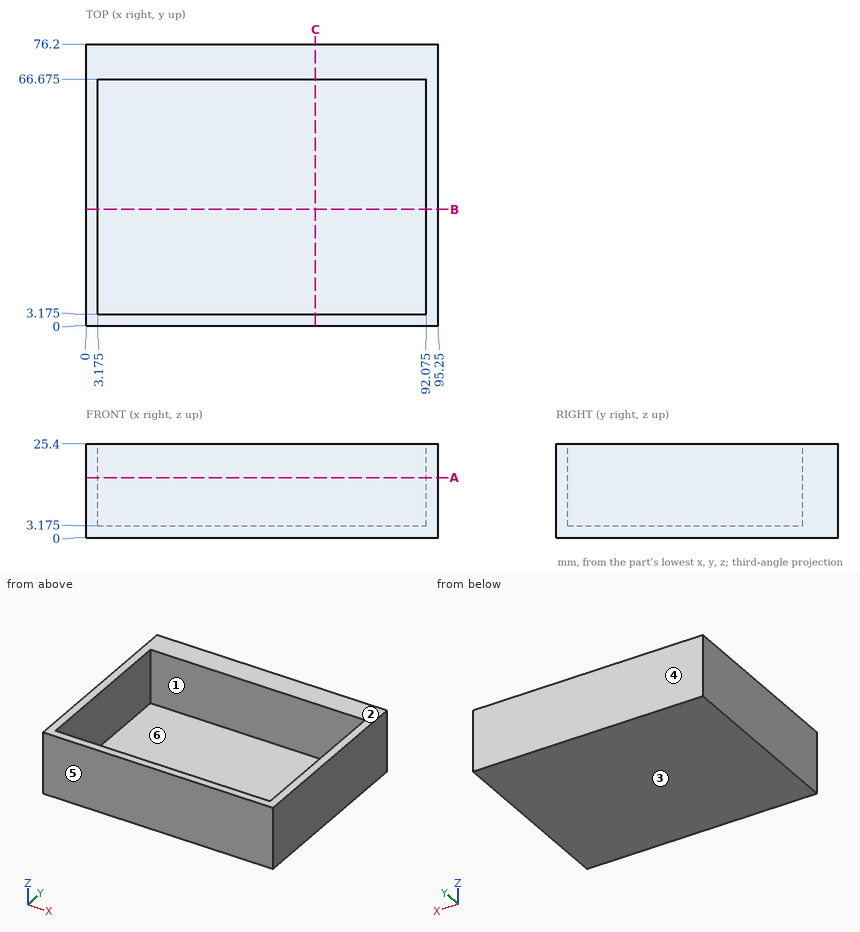
Can you work these out from the drawing? Everything is in mm from the part's minimum corner. A direction names the side the tool comes from. Round coordinates to 2 decimals unless told otherwise and drop trailing zeros. Loops run counter-clockwise (first coordinate to the right, second up) from the corner with the lowest first, then second, coordinate; pieces in that order, holes last. Notation, with made-up numbers: (20, 57) - (57, 57) arc R23 ccw to (57, 71) - close; hole circle Ø4 at (11, 15.25). An arc over 180 degrees is marked (long way). Answer as CSV lines item,"result".
1. I want a section at A-A on z = 16.25. List the corners of the cut face in (x, y) for me (3 decimals), then the cut area to 3 significant figures.
Filled in:
outline,"(0, 0) - (95.25, 0) - (95.25, 76.2) - (0, 76.2) - close; hole (3.175, 3.175) - (92.075, 3.175) - (92.075, 66.675) - (3.175, 66.675) - close"
area,"1,610 mm^2"
2. Please list where these lines run through material, in increasing order: line 1 along X through (y, z) = (5, 13) (3 decimals); line 2 along Y through (x, z) = (57, 5.25) (3 decimals); line 3 along Z through (x, y) = (87, 51) (3 decimals). Write a range as [from, to].
Filled in:
line 1,"x = [0, 3.175], [92.075, 95.25]"
line 2,"y = [0, 3.175], [66.675, 76.2]"
line 3,"z = [0, 3.175]"
3. On a 3-axis mill with a long thin cutter (end or side, diameter ignored), from which of +Z, -Z, +X, -X, +Y, -Y can I reach the whole of each face in a straight line? I mean the marked faces 1 and 2. Say none if no direction works.
Filled in:
face 1,"+Z"
face 2,"+Z, +X, -X, +Y, -Y"
4. I want a section at B-B on y = 31.5. List the corners of the cut face in (x, z) for me (3 decimals), then the cut area to 3 significant figures.
Filled in:
outline,"(0, 0) - (95.25, 0) - (95.25, 25.4) - (92.075, 25.4) - (92.075, 3.175) - (3.175, 3.175) - (3.175, 25.4) - (0, 25.4) - close"
area,"444 mm^2"
5. I want a section at C-C on x = 62. List the corners of the cut face in (y, z) for me (3 decimals).
Filled in:
outline,"(0, 0) - (76.2, 0) - (76.2, 25.4) - (66.675, 25.4) - (66.675, 3.175) - (3.175, 3.175) - (3.175, 25.4) - (0, 25.4) - close"
6. For pin 1 Ø8 at (x, y) = (45.5, 40) entering from +Z (3 decimals); pin 2 Ø2 at (x, z) = (70, 9) entering from -Y, each with a flat end and sliding along its axis, tell me the tip position at first contact or that it passes through.
Filled in:
pin 1,"stops at z = 3.175"
pin 2,"stops at y = 0"
7. We'd pull the mould along Y, two halves only. Please class the marked faces 3, 4, 5 and 6: +Y half, -Y half, draft (parallel to the pull), parting line (faces both ways), or undercut.
Filled in:
face 3,"draft"
face 4,"+Y half"
face 5,"-Y half"
face 6,"undercut"
